from build123d import *

# Parameters (mm, degrees)
SKETCH1_R           = 83
SKETCH1_R_2         = 12.5
BOSS_EXTRUDE1_DEPTH = 7
SKETCH14_R          = 2
CUT_EXTRUDE2_DEPTH  = 133
CUT_EXTRUDE3_DEPTH  = 3.3
SKETCH16_R          = 2.5
CUT_EXTRUDE4_DEPTH  = 10


with BuildPart() as part:
    # Sketch1 → Boss-Extrude1 (new body)
    with BuildSketch(Plane(origin=(0, 0, 0), x_dir=(1, 0, 0), z_dir=(0, 1, 0))):
        with Locations(Location((0, 0, 0), (0, 0, 270))):
            Circle(SKETCH1_R)
        with Locations(Location((0, 40, 0), (0, 0, 270))):
            Circle(SKETCH1_R_2, mode=Mode.SUBTRACT)
        with Locations(Location((0, -40, 0), (0, 0, 270))):
            Circle(SKETCH1_R_2, mode=Mode.SUBTRACT)
    extrude(amount=BOSS_EXTRUDE1_DEPTH)

    # Sketch14 → Cut-Extrude2 (cut)
    with BuildSketch(Plane(origin=(0, 7, 0), x_dir=(1, 0, 0), z_dir=(0, 1, 0))):
        with Locations(Location((-53.033008589, 53.033008589, 0), (0, 0, 270))):
            Circle(SKETCH14_R)
        with Locations(Location((53.033008589, 53.033008589, 0), (0, 0, 270))):
            Circle(SKETCH14_R)
        with Locations(Location((53.033008589, -53.033008589, 0), (0, 0, 270))):
            Circle(SKETCH14_R)
        with Locations(Location((-53.033008589, -53.033008589, 0), (0, 0, 270))):
            Circle(SKETCH14_R)
    extrude(amount=-CUT_EXTRUDE2_DEPTH, mode=Mode.SUBTRACT)

    # Sketch15 → Cut-Extrude3 (cut)
    with BuildSketch(Plane(origin=(0, 7, 0), x_dir=(1, 0, 0), z_dir=(0, 1, 0))):
        Polygon((-49.533008589, 55.053734531), (-53.033008589, 57.074460473), (-56.533008589, 55.053734531), (-56.533008589, 51.012282647), (-53.033008589, 48.991556705), (-49.533008589, 51.012282647), align=None)
        Polygon((55.053734531, 49.533008589), (57.074460473, 53.033008589), (55.053734531, 56.533008589), (51.012282647, 56.533008589), (48.991556705, 53.033008589), (51.012282647, 49.533008589), align=None)
        Polygon((49.533008589, -55.053734531), (53.033008589, -57.074460473), (56.533008589, -55.053734531), (56.533008589, -51.012282647), (53.033008589, -48.991556705), (49.533008589, -51.012282647), align=None)
        Polygon((-55.053734531, -49.533008589), (-57.074460473, -53.033008589), (-55.053734531, -56.533008589), (-51.012282647, -56.533008589), (-48.991556705, -53.033008589), (-51.012282647, -49.533008589), align=None)
    extrude(amount=-CUT_EXTRUDE3_DEPTH, mode=Mode.SUBTRACT)

    # Sketch16 → Cut-Extrude4 (cut)
    with BuildSketch(Plane(origin=(0, 7, 0), x_dir=(1, 0, 0), z_dir=(0, 1, 0))):
        with Locations(Location((-40, 0, 0), (0, 0, 270))):
            Circle(SKETCH16_R)
        with Locations(Location((40, 0, 0), (0, 0, 270))):
            Circle(SKETCH16_R)
        with Locations(Location((0, 0, 0), (0, 0, 270))):
            Circle(SKETCH16_R)
    extrude(amount=-CUT_EXTRUDE4_DEPTH, mode=Mode.SUBTRACT)


solid = part.part
The listing builds one solid part. Answer for the finished solid, in the listing's coordinates (mm). A direction names the side the tool comes from. Coordinates: 2 decimals unless noted, no trailing zeros. Write each loop counter-clockwise with the first axis right and the second up, starting at its lowest first coordinate (ties: lowest second). Pieces come first, ordered by that corner, then holes. Notation, with made-up numbers: M -1,46 L 37,46 A13 ccw 37,63 Z; hole C 55.25,19.25 d7. An arc over 180 degrees is marked long. Put each result on its own line as item: value. Start each with the question number.
1. Consider line 1 (X direction, y = 5.75, z = 0); line 2 (Z direction, x = -8, y = 1.5); line 3 (X direction, y = 1.25, z = -43). Determine where each line is inside the solid, lowest interval first. Write a range as from..to.
2. Which of the six approach directions +Z, -Z, +X, -X, +Y, -Y give full straight-line access (tool end or side, diameter ignored) to faces 1 (the flat face through (55, 3.7, -55)), 2 (the cylindrical face through (8.45, 3.45, -49.21))?
3. A cutting plane is placed at B-B on z = 0. Write down the section's boundary in (x, y), then the cut area to 3 significant figures.
4. A cutting plane is placed at D-D on x = 40. Write down the section's boundary in (y, z), then the cut area to 3 significant figures.
5. A cutting plane is placed at A-A on y = 5. Count the separate pieces of the cut face and the enclosed holes in it, then the cut area to 3 significant figures.
6. Flat-ended cylindrical pins translate along their axes: P1, Ø2.5, axis at y = 6, z = 53, coming from the +X side; P2, Ø1.6, axis at y = 5.5, z = 53, coming from the -X side; P3, Ø4, axis at x = 16.5, y = 5, coming from the +Z side; P4, Ø1, axis at x = -7.5, z = -10, coming from the -Y side. Find the tip coordinate at first contact, or state that the pin passes through.
7. For a pull along X with two mould halves and no side action, classify faces 3 (the cylindrical face through (24.931, 3.451, 79.167)), 4 (the flat face through (-17, 7, -1)), 5 (the flat face through (-51, 3.7, 51)) as pulls with the +X half, pulls with the -X half, needs draft (parallel to the pull), parting line crosses it, or undercut.
8. A cutting plane is placed at C-C on z = 40. Write down the section's boundary in (x, y).
Resolved:
1. line 1: x = -83..-42.5, -37.5..-2.5, 2.5..37.5, 42.5..83
1. line 2: z = -82.61..-49.6, -30.4..30.4, 49.6..82.61
1. line 3: x = -70.99..-12.13, 12.13..70.99
2. face 1: +Y
2. face 2: +Y, -Y
3. outline: M -83,0 L -42.5,0 L -42.5,7 L -83,7 Z; M -37.5,0 L -2.5,0 L -2.5,7 L -37.5,7 Z; M 2.5,0 L 37.5,0 L 37.5,7 L 2.5,7 Z; M 42.5,0 L 83,0 L 83,7 L 42.5,7 Z
3. area: 1,060 mm2
4. outline: M 0,-72.73 L 7,-72.73 L 7,-2.5 L 0,-2.5 Z; M 0,2.5 L 7,2.5 L 7,72.73 L 0,72.73 Z
4. area: 983 mm2
5. separate pieces: 1
5. enclosed holes: 9
5. area: 20,400 mm2
6. P1: stops at x = 64.89
6. P2: stops at x = -64.53
6. P3: stops at z = 81.72
6. P4: stops at y = 0
7. face 3: parting line crosses it
7. face 4: needs draft
7. face 5: undercut
8. outline: M -72.73,0 L -12.5,0 L -12.5,7 L -72.73,7 Z; M 12.5,0 L 72.73,0 L 72.73,7 L 12.5,7 Z
